Input: part model. Units: mm. Frame: model coordinates. A direction names the side the tool comes from. Round coordinates to 2 decimals unless told otherwise and drop trailing zeros. Loops run counter-clockwise (first coordinate to the right, second up) from the corner with the lowest first, then second, coordinate; pieces in that order, holes last. Notation, with made-up numbers: (62, -11) - (99, -11) arc R8 ccw to (99, -6) - close; hole circle Ø4 at (33.5, -10). An arc over 180 degrees is marked (long way). One line per question, with ' | ' between items. Start each with the question number.
from build123d import *

# Parameters (mm, degrees)
SKETCH1_R          = 34.5
SKETCH1_R_2        = 5
BASE_EXTRUDE_DEPTH = 20


with BuildPart() as part:
    # Sketch1 → Base-Extrude (new body)
    with BuildSketch(Plane.XY):
        with Locations((255.493849666, -76.580612243)):
            Circle(SKETCH1_R)
        with Locations((255.493849666, -76.580612243)):
            Circle(SKETCH1_R_2, mode=Mode.SUBTRACT)
        with BuildLine():
            Line((268.439049892, -83.080585027), (278.355348881, -84.08056418))
            ThreePointArc((278.355348881, -84.08056418), (266.908732596, -97.760741447), (249.188294551, -99.799944708))
            Line((249.188294551, -99.799944708), (253.805371583, -90.9673039))
            ThreePointArc((253.805371583, -90.9673039), (262.366151463, -89.332056204), (268.439049892, -83.080585027))
        make_face(mode=Mode.SUBTRACT)
        with BuildLine():
            Line((242.946837579, -83.819420347), (236.659216854, -91.552386762))
            ThreePointArc((236.659216854, -91.552386762), (231.469396076, -75.2679603), (238.402528058, -59.645909673))
            Line((238.402528058, -59.645909673), (243.810204365, -68.0178856))
            ThreePointArc((243.810204365, -68.0178856), (241.029987303, -75.790333415), (242.946837579, -83.819420347))
        make_face(mode=Mode.SUBTRACT)
        with BuildLine():
            Line((251.755601813, -52.812504863), (255.382868286, -62.095601431))
            ThreePointArc((255.382868286, -62.095601431), (263.051568152, -64.223074204), (268.439022561, -70.080585027))
            Line((268.439022561, -70.080585027), (278.355317346, -69.08056418))
            ThreePointArc((278.355317346, -69.08056418), (268.047208684, -56.054760182), (251.755601813, -52.812504863))
        make_face(mode=Mode.SUBTRACT)
    extrude(amount=BASE_EXTRUDE_DEPTH)


solid = part.part
(1) Pull-direction query (X, two-part tool) for faces 3 (the face through (221.027, -75.064, 9.86)), 4 (the face through (273.328, -69.588, 9.86)), 5 (the face through (255, -84, 0)); classes: released by +X, released by -X, zero draft, split by the parting line, or undercut.
(2) Reachability of faces 1 (the face through (255, -84, 20)), 2 (the face through (239.85, -87.63, 9.86)) from +Z, -Z, +X, -X, +Y, -Y: full face, straight path, thin tool, end or side. Return the list, or none.
(3) Line query: line 1 along X through (y, z) = (-60, 3); line 2 along Y through (x, z) = (270, 18); line 3 along X through (y, z) = (-89.5, 2). Output: solid intervals per line, ascending. Write a range as from..to.
(4) Section C-C, the plane x = 277.5. Output: boundary loops of the cut face in (y, z), plus the area to 3 significant figures.
(5) Section D-D, the plane z = 12. Output: boundary loops of the cut face in (x, y).
(6) Section B-B, the plane y = -73. Output: boundary loops of the cut face in (x, z), plus the area to 3 significant figures.
(7) Section A-A, the plane x = 239.5. Output: boundary loops of the cut face in (y, z), plus the area to 3 significant figures.
(8) Pin query (flat end, axial travel): P1, Ø3, axis at y = -72.5, z = 12, coming from the -X side; P2, Ø1.5, axis at x = 233.5, z = 4, coming from the -Y side; P3, Ø4, axis at y = -87, z = 15, coming from the -X side; P4, Ø8, axis at x = 255.49, y = -76.58, coming from the -Z side. Return the tip coordinate at first contact, or that it passes through.
Derived:
1) face 3: split by the parting line | face 4: undercut | face 5: zero draft
2) face 1: +Z, +X, -X, +Y, -Y | face 2: +Z, -Z
3) line 1: x = 225.24..238.06, 238.63..254.56, 272.93..285.75 | line 2: y = -107.88..-95.78, -83.24..-69.92, -57.39..-45.28 | line 3: x = 223.5..235.2, 238.33..262.04, 275.79..287.48
4) outline: (-103.15, 0) - (-86.31, 0) - (-86.31, 20) - (-103.15, 20) - close; (-83.99, 0) - (-69.17, 0) - (-69.17, 20) - (-83.99, 20) - close; (-66.85, 0) - (-50.01, 0) - (-50.01, 20) - (-66.85, 20) - close | area: 970 mm²
5) outline: circle Ø69 at (255.49, -76.58); hole (236.66, -91.55) - (242.95, -83.82) arc R14.49 cw to (243.81, -68.02) - (238.4, -59.65) arc R24.06 ccw to start; hole (249.19, -99.8) arc R24.06 ccw to (278.36, -84.08) - (268.44, -83.08) arc R14.49 cw to (253.81, -90.97) - close; hole circle Ø10 at (255.49, -76.58); hole (251.76, -52.81) - (255.38, -62.1) arc R14.49 cw to (268.44, -70.08) - (278.36, -69.08) arc R24.06 ccw to start
6) outline: (221.18, 0) - (231.7, 0) - (231.7, 20) - (221.18, 20) - close; (241.46, 0) - (252, 0) - (252, 20) - (241.46, 20) - close; (258.98, 0) - (289.81, 0) - (289.81, 20) - (258.98, 20) - close | area: 1,040 mm²
7) outline: (-107.15, 0) - (-88.06, 0) - (-88.06, 20) - (-107.15, 20) - close; (-61.34, 0) - (-46.01, 0) - (-46.01, 20) - (-61.34, 20) - close | area: 688 mm²
8) P1: stops at x = 221.09 | P2: stops at y = -103.76 | P3: stops at x = 222.04 | P4: passes through
